CAD build for the part. Positions are in the model's coordinates, mm. Face numbers are marked on the shaded views. Round coordinates to 2 decimals unless told otherwise and drop trailing zeros. Loops run counter-clockwise (first coordinate to the right, second up) from the corner with the lowest first, then second, coordinate; pieces in that order, holes last. Notation, with made-up numbers: (43.5, 23) - (101.5, 23) arc R27 cw to (101.5, 44) - close; hole circle Ø11 at (-26, -8.5). An arc over 180 degrees is marked (long way). Use one line per item in the form item = value.
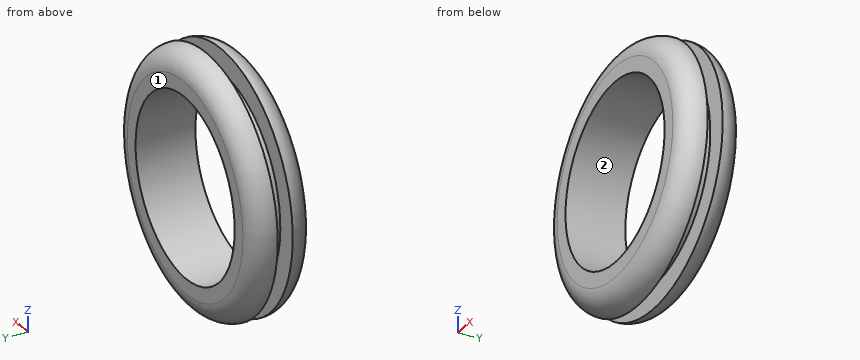
from build123d import *


with BuildPart() as part:
    # Sketch2 → Revolve1 (revolve)
    with BuildSketch(Plane(origin=(0, 0, 0), x_dir=(0, 0, -1), z_dir=(1, 0, 0)), mode=Mode.PRIVATE) as revolve1_sk:
        with BuildLine():
            Line((-19.05, -6.35), (-19.05, 6.35))
            Line((-19.05, 6.35), (-22.225, 6.35))
            ThreePointArc((-22.225, 6.35), (-25.592596045, 4.955096045), (-26.9875, 1.5875))
            Line((-26.9875, 1.5875), (-22.225, 1.5875))
            Line((-22.225, 1.5875), (-22.225, -1.5875))
            Line((-22.225, -1.5875), (-26.9875, -1.5875))
            ThreePointArc((-26.9875, -1.5875), (-25.592596045, -4.955096045), (-22.225, -6.35))
            Line((-22.225, -6.35), (-19.05, -6.35))
        make_face()
    revolve(revolve1_sk.sketch.rotate(Axis((0, -6.35, 0), (0, 1, 0)), 180), axis=Axis((0, -6.35, 0), (0, 1, 0)))


solid = part.part
1) Slice it at C-C (y = -5.25). Write the cut outline in (x, z), plus the area to 3 significant figures.
Report:
outline = circle Ø50.54 at (0, 0); hole circle Ø38.1 at (0, 0)
area = 866 mm^2
2) Drill centre lines: probe 1 along X at (y, z) = (1.5, 0) (3 decimals); probe 2 along Y at (x, z) = (-19.5, 11); probe 3 along X at (y, z) = (-0.25, -13). Where is each one in solid material? Low to high.
Report:
probe_1 = -22.225 to -19.05, 19.05 to 22.225
probe_2 = -6.35 to -1.59, 1.59 to 6.35
probe_3 = -18.03 to -13.92, 13.92 to 18.03
3) Two-plate mould, pull along X, no slides. Class the marked faces 1 and 2: +X half, -X half, draft (parallel to the pull), parting line (faces both ways), or undercut.
Report:
face_1 = draft
face_2 = undercut
4) Slice it at D-D (y = -2.5). Write the cut outline in (x, z), plus the area to 3 significant figures.
Report:
outline = circle Ø53.8 at (0, 0); hole circle Ø38.1 at (0, 0)
area = 1,130 mm^2
5) Flat gauge pins, fed straight in: pin 1 (2 mm diameter, centred on y = -1.5, z = 5, fed in from +X); pin 2 (2 mm diameter, centred on x = -14.5, y = 3.5, fed in from -Z); pin 3 (16 mm diameter, centred on x = 1, z = -4, fed in from +Y); pin 4 (6 mm diameter, centred on x = -6, y = 3.5, fed in from +Z). Where does each tip first touch, or does it go through?
Report:
pin_1 = 26.69
pin_2 = -23.04
pin_3 = through
pin_4 = 26.75
